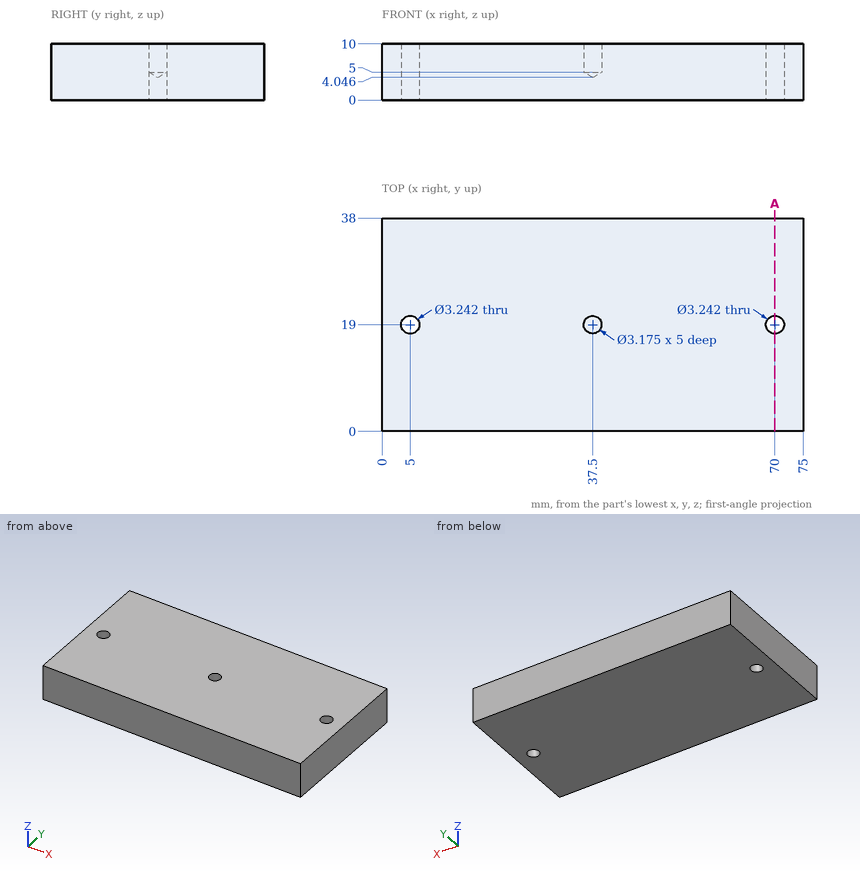
Job drawing, mm, ordinate dimensions from the low corner. One solid piece. Give positions to 0.01 mm unless a question says otherwise; leave off trailing zeros. Order: outer loops, then holes, each group sorted by start corner. A loop starts at its lowest first (then second) coordinate and runs counter-clockwise, first axis right, second up. Notation, with made-up numbers: M -20,78.25 L 25,78.25 A26 cw 25,102.25 Z; hole C 89,-37.5 d6. An arc over 180 degrees is marked long. Put each result on its own line as item: value. Start each with the question number.
(1) Pin check, flat tips, straight feed: pin 1 Ø4 at (x, y) = (70, 19) entering from -Z; pin 2 Ø3 at (x, y) = (5, 19) entering from +Z. Stop position of each tip, or through.
(2) Drill centre lines: L1, parallel to X at y = 19, z = 8; L2, parallel to X at y = 19, z = 4.75; L3, parallel to Y at x = 5, z = 4. Where is each one in solid material? Low to high. Write a range as [from, to].
(3) Band-saw the part on A-A on x = 70. Give the cut face in (y, z).
Results below:
1. pin 1: stops at z = 0
1. pin 2: passes through
2. L1: x = [0, 3.38], [6.62, 35.91], [39.09, 68.38], [71.62, 75]
2. L2: x = [0, 3.38], [6.62, 36.33], [38.67, 68.38], [71.62, 75]
2. L3: y = [0, 17.38], [20.62, 38]
3. outline: M 0,0 L 17.38,0 L 17.38,10 L 0,10 Z; M 20.62,0 L 38,0 L 38,10 L 20.62,10 Z
